Read the model definition and answer for the solid it produces. Units are mm, in the model's axes. A direction names the side the tool comes from. Round coordinates to 2 decimals unless told otherwise and drop trailing zeros. Order: outer loops, then holes, each group sorted by start corner. A loop starts at its lowest first (then second) coordinate and runs counter-clockwise, first axis right, second up.
Autodesk Inventor part; units mm, degrees
ref_plane "Work Plane1" through (0, 23.8125, 0) normal (0, -1, 0) x (1, 0, 0)
ref_plane "YZ Plane" through (0, 0, 0) normal (1, 0, 0) x (0, 1, 0)
ref_plane "XZ Plane" through (0, 0, 0) normal (0, 1, 0) x (-1, 0, 0)
sketch "Sketch1" plane through (0, 0, 0) normal (0, 0, 1) x (1, 0, 0)
  circle A0 centre (0, 0) radius 23.8125
  circle A1 centre (0, 0) radius 6.35
  line L0 (-1.5875, 4.7625) -> (1.5875, 4.7625)
  line L1 (1.5875, 4.7625) -> (1.5875, 7.9375)
  line L2 (1.5875, 7.9375) -> (-1.5875, 7.9375)
  line L3 (-1.5875, 7.9375) -> (-1.5875, 4.7625)
  dimension "d0" = 47.625
  dimension "d1" = 12.7
  dimension "d2" = 3.175
  dimension "d3" = 1.5875
  dimension "d4" = 7.9375
extrude "Extrusion1" add sketch "Sketch1" along normal blind 12.7
ref_plane "Work Plane1" through (0, 23.8125, 0) normal (0, -1, 0) x (1, 0, 0)
sketch "Sketch2" plane through (0, 23.8125, 0) normal (0, -1, 0) x (1, 0, 0)
  circle A0 centre (0, 6.35) radius 1.7272
  line L0 (-23.8125, 12.7) -> (23.8125, 12.7)
  line L1 (-23.8125, 0) -> (23.8125, 0)
  line L2 (-23.8125, 0) -> (-23.8125, 12.7)
  line L3 (23.8125, 0) -> (23.8125, 12.7)
  point P0 (0, 0)
  dimension "d7" = 3.4544
  dimension "d8" = 6.35
  dimension "d9" = 23.8125
extrude "Extrusion2" cut sketch "Sketch2" along normal blind 25.4 contours A0
properties part number "8 ball roller plug"
Q1. A cutting plane is placed at B-B, the plane y = 0. Give the vertices of the cut face in (x, z), plus the area to 3 significant figures.
Outcome:
outline: (-23.81, 0) - (-6.35, 0) - (-6.35, 12.7) - (-23.81, 12.7) - close; (6.35, 0) - (23.81, 0) - (23.81, 12.7) - (6.35, 12.7) - close
area: 444 mm2
Q2. A cutting plane is placed at A-A, the plane x = 0. Give the vertices of the cut face in (y, z), plus the area to 3 significant figures.
Outcome:
outline: (-23.81, 0) - (-6.35, 0) - (-6.35, 12.7) - (-23.81, 12.7) - close; (7.94, 0) - (23.81, 0) - (23.81, 4.62) - (7.94, 4.62) - close; (7.94, 8.08) - (23.81, 8.08) - (23.81, 12.7) - (7.94, 12.7) - close
area: 369 mm2
Q3. For faces 1 (the face through (1.647, 15.085, 5.831)), 2 (the face through (5, -5, 0)), 3 (the face through (0, 7.938, 2)), determine the directions among +Z, -Z, +X, -X, +Y, -Y from which every point of the face is accessible in a straight line to the end or side of a thin tool.
Outcome:
face 1: +Y
face 2: -Z, +X, -X, +Y, -Y
face 3: +Z, -Z
Q4. Straight lines are drawn through the part: probe 1 along Z at (x, y) = (0, 14.5); probe 2 along Y at (x, z) = (0, 9.5); probe 3 along Z at (x, y) = (-1.5, 11). For each, find the intervals that lie inside material, in ascending order.
Outcome:
probe 1: z = 0 to 4.62, 8.08 to 12.7
probe 2: y = -23.81 to -6.35, 7.94 to 23.81
probe 3: z = 0 to 5.49, 7.21 to 12.7
Q5. For a pull along Y with two mould halves and no side action, classify faces 4 (the face through (5, -5, 12.7)), 5 (the face through (1.588, 7, 3)), 6 (the face through (-18.897, 14.49, 6.261)), 7 (the face through (-1.588, 7, 10)) as released by +Y, released by -Y, zero draft, split by the parting line, or undercut.
Outcome:
face 4: zero draft
face 5: undercut
face 6: split by the parting line
face 7: undercut
Q6. Flat-ended cylindrical pins translate along their axes: pin 1 (3.5 mm diameter, centred on x = -0.5, z = 11, fed in from -Y); pin 2 (1 mm diameter, centred on y = -11.5, z = 11, fed in from +X); pin 3 (2 mm diameter, centred on y = 7.5, z = 10, fed in from +X); pin 4 (7.5 mm diameter, centred on x = 0, y = 0, fed in from +Z). Find the tip coordinate at first contact, or state that the pin passes through.
Outcome:
pin 1: stops at y = -23.81
pin 2: stops at x = 21.12
pin 3: stops at x = 22.91
pin 4: passes through
Q7. A cutting plane is placed at D-D, the plane y = 19. Give the vertices of the cut face in (x, z), plus the area to 3 significant figures.
Outcome:
outline: (-14.35, 0) - (14.35, 0) - (14.35, 12.7) - (-14.35, 12.7) - close; hole circle Ø3.45 at (0, 6.35)
area: 355 mm2
